```python
from build123d import *

# Parameters (mm, degrees)
F0_W     = 152.4
F0_H     = 152.4
F1_DEPTH = 25.4
F2_W     = 12.7
F2_H     = 152.4
F3_DEPTH = 101.6
F5_D     = 20.4216
F5_DEPTH = 12.7
F5_TIP   = 6.1352676088
F7_D     = 5
F7_DEPTH = 25.4
F7_TIP   = 1.5021515476
F8_D     = 12.7
F8_DEPTH = 12.7
F8_TIP   = 3.8154649308
F9_D     = 9.525
F9_DEPTH = 44.45
F9_START = 31.75
F9_TIP   = 2.8615986981


with BuildPart() as f1:
    # F0 (on Top) → F1 (new body)
    with BuildSketch(Plane.XY):
        Rectangle(F0_W, F0_H)
    extrude(amount=F1_DEPTH)

    # F2 (on face) → F3 (join)
    with BuildSketch(Plane.XY.offset(25.4)):
        with Locations((-15.875, 0)):
            Rectangle(F2_W, F2_H)
        with Locations((15.875, 0)):
            Rectangle(F2_W, F2_H)
    extrude(amount=F3_DEPTH)

    # F5
    with Locations(Plane.YZ.offset(22.225)):
        with Locations((0, 65.4)):
            Hole(F5_D / 2, depth=F5_DEPTH)
            with Locations((0, 0, -(F5_DEPTH + F5_TIP / 2))):  # 118° drill point
                Cone(0, F5_D / 2, F5_TIP, mode=Mode.SUBTRACT)

    # F7
    with Locations(Plane(origin=(0, 0, 0), x_dir=(1, 0, 0), z_dir=(0, 0, -1))):
        with Locations((1.525, 0)):
            Hole(F7_D / 2, depth=F7_DEPTH)
            with Locations((0, 0, -(F7_DEPTH + F7_TIP / 2))):  # 118° drill point
                Cone(0, F7_D / 2, F7_TIP, mode=Mode.SUBTRACT)

    # F8
    with Locations(Plane(origin=(0, 0, 0), x_dir=(1, 0, 0), z_dir=(0, 0, -1))):
        with Locations((1.525, 0)):
            Hole(F8_D / 2, depth=F8_DEPTH)
            with Locations((0, 0, -(F8_DEPTH + F8_TIP / 2))):  # 118° drill point
                Cone(0, F8_D / 2, F8_TIP, mode=Mode.SUBTRACT)

    # F9
    # its depths count from where the whole tool has entered the part; down to there all is cleared
    with Locations(Plane.YZ.offset(22.225).offset(-F9_START)):
        with Locations((0, 65.4)):
            Hole(F9_D / 2, depth=F9_DEPTH)
            with Locations((0, 0, -(F9_DEPTH + F9_TIP / 2))):  # 118° drill point
                Cone(0, F9_D / 2, F9_TIP, mode=Mode.SUBTRACT)


solid = f1.part
```
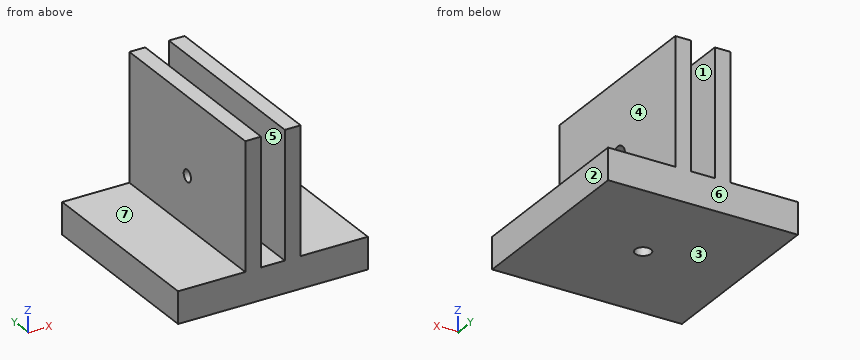
Can you work these out from the model? Positions are in its coordinate system, mm. Face numbers are marked on the shaded views. A direction names the side the tool comes from. Give positions to 0.01 mm unless a question says otherwise; leave off trailing zeros. Loops run counter-clockwise (first coordinate to the right, second up) from the corner with the lowest first, then second, coordinate; pieces in that order, holes last. Notation, with made-up numbers: M 74,2.25 L 99,2.25 A24 cw 99,26.25 Z; hole C 4,-16.5 d10. An arc over 180 degrees is marked long. Answer in a Markdown table with one row per item.
1. For pin 1 Ø9.5 at (x, y) = (-4, 18) entering from +Z; pin 2 Ø7.5 at (y, z) = (0, 65.4) entering from -X; pin 3 Ø23.5 at (y, z) = (0, 65.4) entering from -X (3 decimals), each with a flat end and sliding along its axis, tell me the tip position at first contact or that it passes through.
Taken from the geometry:
| item | result |
|---|---|
| pin 1 | stops at z = 25.4 |
| pin 2 | passes through |
| pin 3 | stops at x = -22.225 |
2. Thinking about a two-plate mould opening in X: for the marked faces 1, 2 and 3, which applies, released by +X, released by -X, zero draft, split by the parting line, or undercut?
Taken from the geometry:
| item | result |
|---|---|
| face 1 | undercut |
| face 2 | released by +X |
| face 3 | zero draft |
3. Suppose I cut it at A-A on z = 49.5. Write out the boundary of the cut face in (x, y) (3 decimals).
Taken from the geometry:
| item | result |
|---|---|
| outline | M -22.225,-76.2 L -9.525,-76.2 L -9.525,76.2 L -22.225,76.2 Z; M 9.525,-76.2 L 22.225,-76.2 L 22.225,76.2 L 9.525,76.2 Z |
4. Suppose I cut it at D-D on y = -62.5. Write out the boundary of the cut face in (x, z) (3 decimals), plus the area to 3 significant figures.
Taken from the geometry:
| item | result |
|---|---|
| outline | M -76.2,0 L 76.2,0 L 76.2,25.4 L 22.225,25.4 L 22.225,127 L 9.525,127 L 9.525,25.4 L -9.525,25.4 L -9.525,127 L -22.225,127 L -22.225,25.4 L -76.2,25.4 Z |
| area | 6,450 mm² |
5. If I drill on line 1 along X through (y, z) = (-22, 85) (3 decimals); line 2 along Y through (x, z) = (19, 65); line 3 along Z through (x, y) = (19.25, 0), over which ranges is the centre line in solid material (lowest first)?
Taken from the geometry:
| item | result |
|---|---|
| line 1 | x = -22.225 to -9.525, 9.525 to 22.225 |
| line 2 | y = -76.2 to -10.2, 10.2 to 76.2 |
| line 3 | z = 0 to 55.19, 75.61 to 127 |
6. Which directions (+Z, -Z, +X, -X, +Y, -Y) give clear straight access to the entire face, cutting with the end or side of a thin tool? Please do the marked faces 4, 5, 6 and 7.
Taken from the geometry:
| item | result |
|---|---|
| face 4 | +Z, +X, +Y, -Y |
| face 5 | +Z, +Y, -Y |
| face 6 | +Z, -Z, +X, -X, +Y |
| face 7 | +Z, -X, +Y, -Y |
7. Suppose I cut it at B-B on y = 0. Write out the boundary of the cut face in (x, z) (1 decimal), plus the area to 3 significant figures.
Taken from the geometry:
| item | result |
|---|---|
| outline | M -76.2,0 L -4.8,0 L -4.8,12.7 L -1,15 L -1,25.4 L -9.5,25.4 L -9.5,60.6 L -22.2,60.6 L -22.2,25.4 L -76.2,25.4 Z; M -22.2,70.2 L -9.5,70.2 L -9.5,127 L -22.2,127 Z; M 4,15 L 7.9,12.7 L 7.9,0 L 76.2,0 L 76.2,25.4 L 22.2,25.4 L 22.2,55.2 L 9.5,55.2 L 9.5,25.4 L 4,25.4 Z; M 9.5,75.6 L 22.2,75.6 L 22.2,127 L 9.5,127 Z |
| area | 5,840 mm² |
8. Suppose I cut it at C-C on z = 65.4. Write out the boundary of the cut face in (x, y) (1 decimal), plus the area to 3 significant figures.
Taken from the geometry:
| item | result |
|---|---|
| outline | M -22.2,-76.2 L -9.5,-76.2 L -9.5,-4.8 L -22.2,-4.8 Z; M -22.2,4.8 L -9.5,4.8 L -9.5,76.2 L -22.2,76.2 Z; M 9.5,-76.2 L 22.2,-76.2 L 22.2,-10.2 L 9.5,-10.2 Z; M 9.5,10.2 L 22.2,10.2 L 22.2,76.2 L 9.5,76.2 Z |
| area | 3,490 mm² |
